The listing builds one solid part. Answer for the finished solid, in the listing's coordinates (mm). A direction names the side the tool comes from. Give positions to 0.01 mm unless a question says otherwise; leave off trailing zeros. Write each loop counter-clockwise with the first axis right and the second up, starting at its lowest first coordinate (ties: lowest second). Pieces come first, ordered by that corner, then holes.
```python
from build123d import *

# Parameters (mm, degrees)
SKETCH1_R               = 9
SKETCH1_R_2             = 5
BOSS_EXTRUDE1_DEPTH     = 30
SKETCH2_W               = 45
SKETCH2_H               = 42
CUT_EXTRUDE2_DEPTH      = 107.324973548
CUT_EXTRUDE3_DEPTH      = 60
CUT_EXTRUDE4_DEPTH      = 113.534439173
CUT_EXTRUDE4_DEPTH_BACK = 113.534439173
SKETCH4_R               = 9
SKETCH4_R_2             = 8
SKETCH5_R               = 13
CUT_EXTRUDE5_DEPTH      = 12
SKETCH6_W               = 40
SKETCH6_H               = 4
CUT_EXTRUDE6_DEPTH      = 133.140077214


with BuildPart() as part:
    # Sketch1 → Boss-Extrude1 (new, symmetric)
    with BuildSketch(Plane.XY):
        with BuildLine():
            Line((0, 0), (0, 6))
            Line((0, 6), (8, 6))
            Line((8, 6), (8, 41.026334039))
            ThreePointArc((8, 41.026334039), (5.77502784, 77.748239349), (38, 60))
            Line((38, 60), (38, 25))
            Line((38, 25), (50, 25))
            Line((50, 25), (50, 12))
            Line((50, 12), (100, 12))
            Line((100, 12), (100, 0))
            Line((100, 0), (0, 0))
        make_face()
        with Locations((17, 60)):
            Circle(SKETCH1_R, mode=Mode.SUBTRACT)
        with Locations((23, 12)):
            Circle(SKETCH1_R_2, mode=Mode.SUBTRACT)
    extrude(amount=BOSS_EXTRUDE1_DEPTH, both=True)

    # Sketch2 → Cut-Extrude2 (cut, through all)
    with BuildSketch(Plane(origin=(38, 0, 0), x_dir=(0, 0, -1), z_dir=(1, 0, 0))):
        with Locations((0, 60)):
            Rectangle(SKETCH2_W, SKETCH2_H)
    extrude(amount=-CUT_EXTRUDE2_DEPTH, mode=Mode.SUBTRACT)

    # Sketch3 → Cut-Extrude3 (cut)
    with BuildSketch(Plane(origin=(0, 12, 0), x_dir=(1, 0, 0), z_dir=(0, 1, 0))):
        with BuildLine():
            ThreePointArc((70, 30), (91.213203436, 21.213203436), (100, 0))
            Line((100, 0), (100, 30))
            Line((100, 30), (70, 30))
        make_face()
        with BuildLine():
            Line((100, -30), (100, 0))
            ThreePointArc((100, 0), (91.213203436, -21.213203436), (70, -30))
            Line((70, -30), (100, -30))
        make_face()
    extrude(amount=-CUT_EXTRUDE3_DEPTH, mode=Mode.SUBTRACT)

    # Sketch4 → Cut-Extrude4 (cut, two sides: drawn at the far end of the back side and taken through both)
    with BuildSketch(Plane(origin=(0, 39, 0), x_dir=(1, 0, 0), z_dir=(0, 1, 0)).offset(-CUT_EXTRUDE4_DEPTH_BACK)):
        with Locations(Location((23, 0, 0), (0, 0, 180))):
            Circle(SKETCH4_R)
        with Locations(Location((70, 0, 0), (0, 0, 180))):
            Circle(SKETCH4_R_2)
    extrude(amount=CUT_EXTRUDE4_DEPTH + CUT_EXTRUDE4_DEPTH_BACK, mode=Mode.SUBTRACT)

    # Sketch5 → Cut-Extrude5 (cut)
    with BuildSketch(Plane(origin=(50, 0, 0), x_dir=(0, 0, -1), z_dir=(1, 0, 0))):
        with Locations((0, 25)):
            Circle(SKETCH5_R)
    extrude(amount=-CUT_EXTRUDE5_DEPTH, mode=Mode.SUBTRACT)

    # Sketch6 → Cut-Extrude6 (cut, through all)
    with BuildSketch(Plane.ZY):
        with Locations((0, 2)):
            Rectangle(SKETCH6_W, SKETCH6_H)
    extrude(amount=-CUT_EXTRUDE6_DEPTH, mode=Mode.SUBTRACT)


solid = part.part
```
Item 1: Determine the mould class of faces 1 (the face through (76.349, 7.944, -4.868)), 2 (the face through (25, 32, 30)), 3 (the face through (8, 23, 0)) for opening direction Z: pulls with the +Z half, pulls with the -Z half, needs draft (parallel to the pull), parting line crosses it, or undercut.
Conclusion:
face 1: undercut
face 2: pulls with the +Z half
face 3: needs draft
Item 2: A cutting plane is placed at B-B, the plane y = 19. Give the vertices of the cut face in (x, z), plus the area to 3 significant figures.
Conclusion:
outline: (8, -30) - (50, -30) - (50, -11.53) - (38, -11.53) - (38, 11.53) - (50, 11.53) - (50, 30) - (8, 30) - close; hole circle Ø18 at (23, 0)
area: 1,990 mm2
Item 3: A cutting plane is placed at A-A, the plane x = 12. Give the vertices of the cut face in (y, z), plus the area to 3 significant figures.
Conclusion:
outline: (0, -30) - (52.52, -30) - (52.52, -22.5) - (39, -22.5) - (39, 22.5) - (52.52, 22.5) - (52.52, 30) - (0, 30) - (0, 20) - (4, 20) - (4, -20) - (0, -20) - close; (67.48, -30) - (80.4, -30) - (80.4, -22.5) - (67.48, -22.5) - close; (67.48, 22.5) - (80.4, 22.5) - (80.4, 30) - (67.48, 30) - close
area: 2,580 mm2
Item 4: Each of these flat-tipped pins is pushed along its axis until it touches: P1, Ø14.5, axis at x = 70, z = 0, coming from the +Y side; P2, Ø2, axis at y = 36, z = -20.5, coming from the -X side; P3, Ø4, axis at y = 18.5, z = 16, coming from the +X side; P4, Ø4, axis at x = 35, z = 15, coming from the +Y side. Where does it stop, or does it pass through?
Conclusion:
P1: passes through
P2: stops at x = 8
P3: stops at x = 50
P4: stops at y = 39
Item 5: A cutting plane is placed at C-C, the plane z = -6. Give the vertices of the cut face in (x, y).
Conclusion:
outline: (0, 4) - (16.29, 4) - (16.29, 39) - (8, 39) - (8, 6) - (0, 6) - close; (29.71, 4) - (64.71, 4) - (64.71, 12) - (50, 12) - (50, 13.47) - (38, 13.47) - (38, 39) - (29.71, 39) - close; (75.29, 4) - (99.39, 4) - (99.39, 12) - (75.29, 12) - close
Item 6: Which of the six approach directions +Z, -Z, +X, -X, +Y, -Y give full straight-line access (tool end or side, diameter ignored) to faces 4 (the face through (46, 2, 20)), 5 (the face through (33, 39, 0)), 6 (the face through (50, 19, -18)), 7 (the face through (4, 6, 0)), 8 (the face through (44, 12, 0))?
Conclusion:
face 4: +X, -X, -Y
face 5: +X, -X, +Y
face 6: +Z, -Z, +X, +Y
face 7: +Z, -Z, -X
face 8: +X, +Y
Item 7: A cutting plane is placed at D-D, the plane x = 43. Give the vertices of the cut face in (y, z), plus the area to 3 significant figures.
Conclusion:
outline: (0, -30) - (25, -30) - (25, -13) arc R13 cw to (25, 13) - (25, 30) - (0, 30) - (0, 20) - (4, 20) - (4, -20) - (0, -20) - close
area: 1,070 mm2
Item 8: Consider probe 1 along Z at (x, y) = (14, 47.5); probe 2 along Y at (x, z) = (23, 25); probe 3 along Z at (x, y) = (28, 26). Determine where each line is inside the solid, lowest interval first.
Conclusion:
probe 1: z = -30 to -22.5, 22.5 to 30
probe 2: y = 0 to 7, 17 to 53.29, 66.71 to 80.12
probe 3: z = -30 to -7.48, 7.48 to 30
